Work out the finished part from the listing and answer in its coordinate system (mm). Face numbers are marked on the shaded views. A direction names the side the tool comes from. Coordinates: 2 decimals unless noted, no trailing zeros. Order: outer loops, then holes, each group sorted by start corner. A loop starts at its lowest first (then second) coordinate and runs counter-clockwise, first axis right, second up.
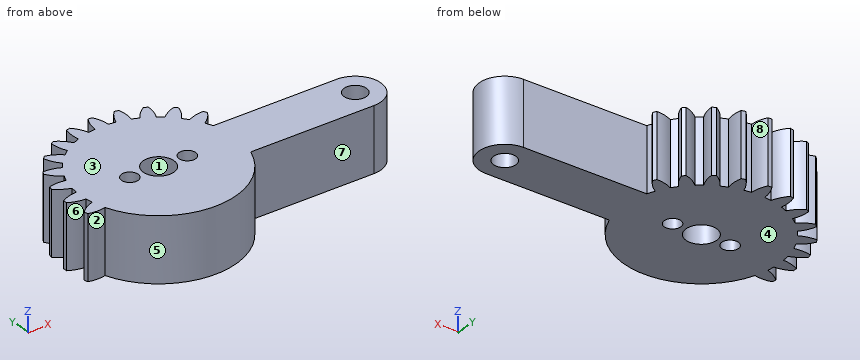
```python
from build123d import *

# Parameters (mm, degrees)
SKETCH1_R           = 1.75
BOSS_EXTRUDE1_DEPTH = 10
SKETCH2_R           = 2.4
SKETCH2_R_2         = 1.3
CUT_EXTRUDE1_DEPTH  = 40.007683858


with BuildPart() as part:
    # Sketch1 → Boss-Extrude1 (new body)
    with BuildSketch(Plane.XY):
        with BuildLine():
            Line((0.31, 14.63), (-0.31, 14.63))
            ThreePointArc((-0.31, 14.63), (-0.832135832, 13.407942292), (-1.04, 12.095371015))
            ThreePointArc((-1.04, 12.095371015), (-1.584587974, 12.036140617), (-2.125949517, 11.952403049))
            ThreePointArc((-2.125949517, 11.952403049), (-2.66644933, 13.166450339), (-3.487085624, 14.211728743))
            Line((-3.487085624, 14.211728743), (-4.085959636, 14.051260935))
            ThreePointArc((-4.085959636, 14.051260935), (-4.274012312, 12.735705136), (-4.135075236, 11.414059435))
            ThreePointArc((-4.135075236, 11.414059435), (-4.645776869, 11.215897525), (-5.147019088, 10.994898568))
            ThreePointArc((-5.147019088, 10.994898568), (-5.983320376, 12.027686554), (-7.046532125, 12.824951657))
            Line((-7.046532125, 12.824951657), (-7.583467875, 12.514951657))
            ThreePointArc((-7.583467875, 12.514951657), (-7.424621916, 11.195550721), (-6.948351928, 9.954898568))
            ThreePointArc((-6.948351928, 9.954898568), (-7.390363748, 9.631309551), (-7.817327814, 9.288109918))
            ThreePointArc((-7.817327814, 9.288109918), (-8.892438027, 10.069255806), (-10.125769107, 10.564175311))
            Line((-10.125769107, 10.564175311), (-10.564175311, 10.125769107))
            ThreePointArc((-10.564175311, 10.125769107), (-10.069255806, 8.892438027), (-9.288109918, 7.817327814))
            ThreePointArc((-9.288109918, 7.817327814), (-9.631309551, 7.390363748), (-9.954898568, 6.948351928))
            ThreePointArc((-9.954898568, 6.948351928), (-11.195550721, 7.424621916), (-12.514951657, 7.583467875))
            Line((-12.514951657, 7.583467875), (-12.824951657, 7.046532125))
            ThreePointArc((-12.824951657, 7.046532125), (-12.027686554, 5.983320376), (-10.994898568, 5.147019088))
            ThreePointArc((-10.994898568, 5.147019088), (-11.215897525, 4.645776869), (-11.414059435, 4.135075236))
            ThreePointArc((-11.414059435, 4.135075236), (-12.735705136, 4.274012312), (-14.051260935, 4.085959636))
            Line((-14.051260935, 4.085959636), (-14.211728743, 3.487085624))
            ThreePointArc((-14.211728743, 3.487085624), (-13.166450339, 2.66644933), (-11.952403049, 2.125949517))
            ThreePointArc((-11.952403049, 2.125949517), (-12.036140617, 1.584587974), (-12.095371015, 1.04))
            ThreePointArc((-12.095371015, 1.04), (-13.407942292, 0.832135832), (-14.63, 0.31))
            Line((-14.63, 0.31), (-14.63, -0.31))
            ThreePointArc((-14.63, -0.31), (-13.407942292, -0.832135832), (-12.095371015, -1.04))
            ThreePointArc((-12.095371015, -1.04), (-12.036140617, -1.584587974), (-11.952403049, -2.125949517))
            ThreePointArc((-11.952403049, -2.125949517), (-13.166450339, -2.66644933), (-14.211728743, -3.487085624))
            Line((-14.211728743, -3.487085624), (-14.051260935, -4.085959636))
            ThreePointArc((-14.051260935, -4.085959636), (-12.735705136, -4.274012312), (-11.414059435, -4.135075236))
            ThreePointArc((-11.414059435, -4.135075236), (0.071680966, -12.139788377), (11.46209405, -4))
            Line((11.46209405, -4), (30.75, -4))
            ThreePointArc((30.75, -4), (34.75, 0), (30.75, 4))
            Line((30.75, 4), (11.46209405, 4))
            ThreePointArc((11.46209405, 4), (11.243133129, 4.579471307), (10.994898568, 5.147019088))
            ThreePointArc((10.994898568, 5.147019088), (12.027686554, 5.983320376), (12.824951657, 7.046532125))
            Line((12.824951657, 7.046532125), (12.514951657, 7.583467875))
            ThreePointArc((12.514951657, 7.583467875), (11.195550721, 7.424621916), (9.954898568, 6.948351928))
            ThreePointArc((9.954898568, 6.948351928), (9.631309551, 7.390363748), (9.288109918, 7.817327814))
            ThreePointArc((9.288109918, 7.817327814), (10.069255806, 8.892438027), (10.564175311, 10.125769107))
            Line((10.564175311, 10.125769107), (10.125769107, 10.564175311))
            ThreePointArc((10.125769107, 10.564175311), (8.892438027, 10.069255806), (7.817327814, 9.288109918))
            ThreePointArc((7.817327814, 9.288109918), (7.390363748, 9.631309551), (6.948351928, 9.954898568))
            ThreePointArc((6.948351928, 9.954898568), (7.424621916, 11.195550721), (7.583467875, 12.514951657))
            Line((7.583467875, 12.514951657), (7.046532125, 12.824951657))
            ThreePointArc((7.046532125, 12.824951657), (5.983320376, 12.027686554), (5.147019088, 10.994898568))
            ThreePointArc((5.147019088, 10.994898568), (4.645776869, 11.215897525), (4.135075236, 11.414059435))
            ThreePointArc((4.135075236, 11.414059435), (4.274012312, 12.735705136), (4.085959636, 14.051260935))
            Line((4.085959636, 14.051260935), (3.487085624, 14.211728743))
            ThreePointArc((3.487085624, 14.211728743), (2.66644933, 13.166450339), (2.125949517, 11.952403049))
            ThreePointArc((2.125949517, 11.952403049), (1.584587974, 12.036140617), (1.04, 12.095371015))
            ThreePointArc((1.04, 12.095371015), (0.832135832, 13.407942292), (0.31, 14.63))
        make_face()
        Circle(SKETCH1_R, mode=Mode.SUBTRACT)
        with Locations((30.75, 0)):
            Circle(SKETCH1_R, mode=Mode.SUBTRACT)
    extrude(amount=BOSS_EXTRUDE1_DEPTH)

    # Sketch2 → Cut-Extrude1 (cut, through all)
    with BuildSketch(Plane.XY.offset(10)):
        Circle(SKETCH2_R)
        with Locations((-4.5, 0)):
            Circle(SKETCH2_R_2)
        with Locations((4.5, 0)):
            Circle(SKETCH2_R_2)
    extrude(amount=-CUT_EXTRUDE1_DEPTH, mode=Mode.SUBTRACT)


solid = part.part
```
1. For the marked faces 4, 5, 6, 7 and 8, determine the directions among +Z, -Z, +X, -X, +Y, -Y from which every point of the face is accessible in a straight line to the end or side of a thin tool.
2. The part is cut by section A-A (x = 12). Determine the outline of the cut face in (y, z), plus the area to 3 significant figures.
3. Consider probe 1 along Y at (x, z) = (0, 5.5); probe 2 along Y at (x, z) = (30.75, 6); probe 3 along X at (y, z) = (-1.5, 1.5). Determine where each line is inside the solid, lowest interval first.
4. The mould has two halves that part along Y. Classify the marked faces 1, 2 and 3: released by +Y, released by -Y, zero draft, split by the parting line, or undercut.
5. The part is cut by section C-C (x = 23). Determine the outline of the cut face in (y, z).
6. The part is cut by section B-B (z = 5.25). Count the separate pieces of the cut face and the enclosed holes in it, plus the area to 3 significant figures.
7. Flat-ended cylindrical pins translate along their axes: pin 1 (2 mm diameter, centred on x = -4.5, y = 0, fed in from +Z); pin 2 (1.5 mm diameter, centred on x = 6.5, z = 7, fed in from +Y); pin 3 (4 mm diameter, centred on y = -7.5, z = 4, fed in from -X); pin 4 (3 mm diameter, centred on x = 20, z = 7, fed in from -Y). Find the tip coordinate at first contact, or state that the pin passes through.
8. The part is cut by section D-D (y = -6.25). Determine the outline of the cut face in (x, z).
Worked out:
1. face 4: -Z, +X, -X, +Y, -Y
1. face 5: +Z, -Z, -Y
1. face 6: +Z, -Z, -X
1. face 7: +Z, -Z, +X, -Y
1. face 8: +Z, -Z, +Y
2. outline: (-4, 0) - (4, 0) - (4, 10) - (-4, 10) - close; (5.95, 0) - (7.56, 0) - (7.56, 10) - (5.95, 10) - close
2. area: 96.1 mm2
3. probe 1: y = -12.14 to -2.4, 2.4 to 14.63
3. probe 2: y = -4 to -1.75, 1.75 to 4
3. probe 3: x = -12.05 to -1.87, 1.87 to 29.85, 31.65 to 34.46
4. face 1: undercut
4. face 2: released by -Y
4. face 3: zero draft
5. outline: (-4, 0) - (4, 0) - (4, 10) - (-4, 10) - close
6. separate pieces: 1
6. enclosed holes: 4
6. area: 648 mm2
7. pin 1: passes through
7. pin 2: stops at y = 12.82
7. pin 3: stops at x = -10.82
7. pin 4: stops at y = -4
8. outline: (-10.41, 0) - (10.41, 0) - (10.41, 10) - (-10.41, 10) - close
